The listing builds one solid part. Answer for the finished solid, in the listing's coordinates (mm). Give positions to 0.01 mm unless a question says otherwise; leave off trailing zeros. Order: outer loops, then holes, each group sorted by start corner. A loop starts at its lowest first (then second) coordinate and runs counter-clockwise, first axis right, second up. Notation, with made-up numbers: (23, -24.75) - (41, -24.75) arc R19 ccw to (41, -17.75) - close; hole circle Ø8 at (21, 17.25). An arc over 180 degrees is marked (long way). Write each question's results on one line, items separated by ' | '. Start each with the question number.
1. Section D-D (x = -15.24) is taken. Give the vertices of the cut face in (y, z) (3 decimals).
2. Section B-B (x = -7.5) is taken. Give the vertices of the cut face in (y, z).
3. Flat-ended cylindrical pins translate along their axes: pin 1 (12 mm diameter, centred on x = -0.5, y = 8.5, fed in from -Z); pin 2 (3 mm diameter, centred on x = 0, y = -15.24, fed in from -Z) (3 decimals); pin 3 (1.5 mm diameter, centred on x = 12.5, z = 98, fed in from +Y); pin 4 (5 mm diameter, centred on x = -13, z = 23.5, fed in from +Y). Find the tip coordinate at first contact, or state that the pin passes through.
4. Find the intervals of material crossed by L1, parallel to Y at x = 0, z = 7 (3 decimals); L2, parallel to Y at x = 0, z = 140; L3, parallel to Z at x = 7, y = 6.5, in increasing order.
5. Section C-C (z = 113) is taken. Give the vertices of the cut face in (x, y) (3 decimals), and give its area (3 significant figures).
from build123d import *

# Parameters (mm, degrees)
SKETCH1_R           = 19.05
SKETCH1_R_2         = 9.525
BOSS_EXTRUDE1_DEPTH = 141.4653
SKETCH2_R           = 1.7526
CUT_EXTRUDE1_DEPTH  = 9.525
CUT_EXTRUDE2_START  = -9.525
SKETCH3_R           = 1.7526
CUT_EXTRUDE2_DEPTH  = 9.525
SKETCH6_R           = 11.1125
CUT_EXTRUDE3_DEPTH  = 5.55625
CUT_EXTRUDE4_START  = -5.55625
SKETCH7_R           = 11.1125
CUT_EXTRUDE4_DEPTH  = 5.55625


with BuildPart() as part:
    # Sketch1 → Boss-Extrude1 (new body)
    with BuildSketch(Plane.XY):
        with Locations(Location((0, 0, 0), (0, 0, 180))):
            Circle(SKETCH1_R)
        with Locations(Location((0, 0, 0), (0, 0, 180))):
            Circle(SKETCH1_R_2, mode=Mode.SUBTRACT)
    extrude(amount=BOSS_EXTRUDE1_DEPTH)

    # Sketch2 → Cut-Extrude1 (cut)
    with BuildSketch(Plane(origin=(0, 0, 0), x_dir=(-1, 0, 0), z_dir=(0, 0, -1))):
        with Locations((0, 15.24)):
            Circle(SKETCH2_R)
        with Locations((15.24, 0)):
            Circle(SKETCH2_R)
        with Locations((0, -15.24)):
            Circle(SKETCH2_R)
        with Locations((-15.24, 0)):
            Circle(SKETCH2_R)
    extrude(amount=-CUT_EXTRUDE1_DEPTH, mode=Mode.SUBTRACT)

    # Sketch3 → Cut-Extrude2 (cut)
    with BuildSketch(Plane.XY.offset(141.4653).offset(CUT_EXTRUDE2_START)):
        with Locations(Location((0, 15.24, 0), (0, 0, 180))):
            Circle(SKETCH3_R)
        with Locations(Location((15.24, 0, 0), (0, 0, 180))):
            Circle(SKETCH3_R)
        with Locations(Location((0, -15.24, 0), (0, 0, 180))):
            Circle(SKETCH3_R)
        with Locations(Location((-15.24, 0, 0), (0, 0, 180))):
            Circle(SKETCH3_R)
    extrude(amount=CUT_EXTRUDE2_DEPTH, mode=Mode.SUBTRACT)

    # Sketch6 → Cut-Extrude3 (cut)
    with BuildSketch(Plane.XY.offset(141.4653)):
        Circle(SKETCH6_R)
    extrude(amount=-CUT_EXTRUDE3_DEPTH, mode=Mode.SUBTRACT)

    # Sketch7 → Cut-Extrude4 (cut)
    with BuildSketch(Plane(origin=(0, 0, 0), x_dir=(-1, 0, 0), z_dir=(0, 0, -1)).offset(CUT_EXTRUDE4_START)):
        with Locations(Location((0, 0, 0), (0, 0, 180))):
            Circle(SKETCH7_R)
    extrude(amount=CUT_EXTRUDE4_DEPTH, mode=Mode.SUBTRACT)


solid = part.part
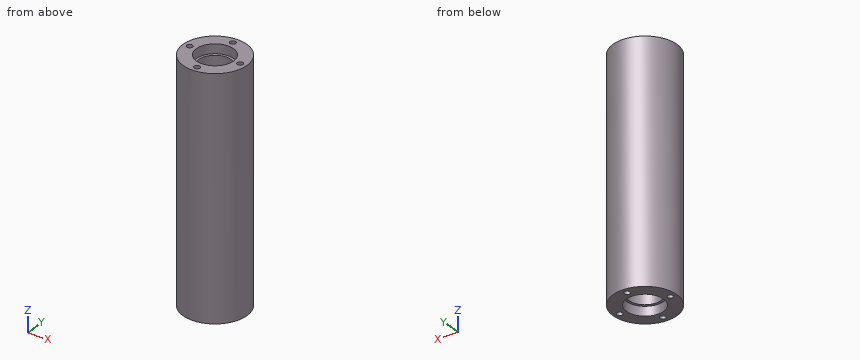
Reported:
1) outline: (-11.43, 0) - (-1.753, 0) - (-1.753, 9.525) - (1.753, 9.525) - (1.753, 0) - (11.43, 0) - (11.43, 141.465) - (1.753, 141.465) - (1.753, 131.94) - (-1.753, 131.94) - (-1.753, 141.465) - (-11.43, 141.465) - close
2) outline: (-17.51, 0) - (-8.2, 0) - (-8.2, 5.56) - (-5.87, 5.56) - (-5.87, 135.91) - (-8.2, 135.91) - (-8.2, 141.47) - (-17.51, 141.47) - close; (5.87, 5.56) - (8.2, 5.56) - (8.2, 0) - (17.51, 0) - (17.51, 141.47) - (8.2, 141.47) - (8.2, 135.91) - (5.87, 135.91) - close
3) pin 1: z = 0 | pin 2: z = 9.525 | pin 3: y = 14.99 | pin 4: y = 15.9
4) L1: -19.05 to -16.993, -13.487 to -9.525, 9.525 to 13.487, 16.993 to 19.05 | L2: -19.05 to -16.99, -13.49 to -11.11, 11.11 to 13.49, 16.99 to 19.05 | L3: 5.56 to 135.91
5) outline: circle Ø38.1 at (0, 0); hole circle Ø19.05 at (0, 0) | area: 855 mm²
